```python
from build123d import *

# Parameters (mm, degrees)
EXTRUDE_1_DEPTH     = 4.8
SKETCH_2_R          = 2
CUT_EXTRUDE_1_DEPTH = 10
CHAMFER_1_SIZE      = 1
CHAMFER_2_SIZE      = 0.75
SKETCH_3_R          = 1.5
EXTRUDE_2_DEPTH     = 1.5
CHAMFER_3_SIZE      = 0.5
FILLET_2_R          = 0.2


with BuildPart() as part:
    # 스케치1 → 보스-돌출1 (new body)
    with BuildSketch(Plane.XY):
        Polygon((0, 0), (20.5, 0), (20.657326787, 1), (21.5, -1.146107212), (21.5, -2.146107212), (16, -2.146107212), (16, -6.5), (5, -6.5), (5, -2), (0, -2), align=None)
    extrude(amount=EXTRUDE_1_DEPTH)

    # 스케치2 → 컷-돌출1 (cut)
    with BuildSketch(Plane.XY.offset(4.8)):
        with Locations((10.5, -3.5)):
            Circle(SKETCH_2_R)
    extrude(amount=-CUT_EXTRUDE_1_DEPTH, mode=Mode.SUBTRACT)

    # 모따기1
    chamfer_1_edges = [part.edges().sort_by_distance(p)[0] for p in [
        (16, -6.5, 2.4),
        (5, -6.5, 2.4),
    ]]
    chamfer(chamfer_1_edges, length=CHAMFER_1_SIZE)

    # 모따기2
    chamfer_2_edges = [part.edges().sort_by_distance(p)[0] for p in [
        (21.5, -2.146107212, 2.4),
        (0, -2, 2.4),
    ]]
    chamfer(chamfer_2_edges, length=CHAMFER_2_SIZE)

    # 스케치3 → 보스-돌출2 (add)
    with BuildSketch(Plane(origin=(0, 0, 0), x_dir=(1, 0, 0), z_dir=(0, 1, 0))):
        with Locations(Location((2.5, -2.4, 0), (0, 0, 90))):
            Circle(SKETCH_3_R)
    extrude(amount=EXTRUDE_2_DEPTH)

    # 모따기3
    chamfer_3_edges = [part.edges().sort_by_distance(p)[0] for p in [
        (2.5, 1.5, 3.9),
    ]]
    chamfer(chamfer_3_edges, length=CHAMFER_3_SIZE)

    # 필렛2
    fillet_2_edges = [part.edges().sort_by_distance(p)[0] for p in [
        (8.5, -3.5, 0),
        (8.5, -3.5, 4.8),
    ]]
    fillet(fillet_2_edges, radius=FILLET_2_R)


solid = part.part
```
Verification items for the finished model (mm, model axes). A direction names the side the tool comes from. Coordinates: 2 decimals unless noted, no trailing zeros. Order: outer loops, then holes, each group sorted by start corner. A loop starts at its lowest first (then second) coordinate and runs counter-clockwise, first axis right, second up. Notation, with made-up numbers: (19.5, 74.25) -> (44.5, 74.25) arc R12 ccw to (44.5, 87.25) -> close; hole circle Ø5 at (-1, 38). An arc over 180 degrees is marked (long way). Put each result on its own line as item: value. Start each with the question number.
1) Cross-section at B-B (y = -3.5). Enter the section's corners in (x, z).
2) Release check for a two-part mould opening along X. For faces 1 (the cylindrical face through (8.9, -4.7, 2.4)), 2 (the flat face through (15.5, -6, 2.4)), 3 (the flat face through (18, -2.146, 2)) record: pulls with the +X half, pulls with the -X half, needs draft (parallel to the pull), parting line crosses it, or undercut.
3) Material ranges on L1, parallel to Y at x = 10.5, z = 2.95; L2, parallel to Y at x = 4.5, z = 4.4; L3, parallel to Y at x = 12.25, z = 1.7, recorded low to high.
4) Cross-section at C-C (z = 2.4). Enter the section's corners in (x, y), plus the area to 3 significant figures.
5) Cross-section at A-A (x = 10.5). Enter the section's corners in (y, z), plus the area to 3 significant figures.
6) Cross-section at D-D (x = 2.5). Enter the section's corners in (y, z).
7) Go/stop test with flat-tipped pins: pin 1 (1.5 mm diameter, centred on x = 14.5, z = 3, fed in from +Y); pin 2 (2.5 mm diameter, centred on y = -3, z = 2.5, fed in from +X); pin 3 (1.5 mm diameter, centred on x = 16, z = 3, fed in from -Y). Record where each tip stops, or that it passes through.
8) Tool access check on faces 4 (the flat face through (20.578, 0.493, 2.366)), 5 (the cylindrical face through (3.075, 0.493, 1.014)), 6 (the flat face through (3, -2, 2)). Record the directions out of +Z, -Z, +X, -X, +Y, -Y that give a thin tool (end or side, any length) a straight path to the whole face; none if there is none.
Geometry check:
1. outline: (5, 0) -> (8.3, 0) arc R0.2 ccw to (8.5, 0.2) -> (8.5, 4.6) arc R0.2 ccw to (8.3, 4.8) -> (5, 4.8) -> close; (12.5, 0.2) arc R0.2 ccw to (12.7, 0) -> (16, 0) -> (16, 4.8) -> (12.7, 4.8) arc R0.2 ccw to (12.5, 4.6) -> close
2. face 1: undercut
2. face 2: pulls with the +X half
2. face 3: needs draft
3. L1: y = -6.5 to -5.5, -1.5 to 0
3. L2: y = -2 to 0
3. L3: y = -6.5 to -4.47, -2.53 to 0
4. outline: (0, -1.25) -> (0.75, -2) -> (5, -2) -> (5, -5.5) -> (6, -6.5) -> (15, -6.5) -> (16, -5.5) -> (16, -2.15) -> (20.75, -2.15) -> (21.5, -1.4) -> (21.5, -1.15) -> (20.66, 1) -> (20.5, 0) -> (4, 0) -> (4, 1) -> (3.5, 1.5) -> (1.5, 1.5) -> (1, 1) -> (1, 0) -> (0, 0) -> close; hole circle Ø4 at (10.5, -3.5)
4. area: 83.4 mm^2
5. outline: (-6.5, 0) -> (-5.7, 0) arc R0.2 ccw to (-5.5, 0.2) -> (-5.5, 4.6) arc R0.2 ccw to (-5.7, 4.8) -> (-6.5, 4.8) -> close; (-1.5, 0.2) arc R0.2 ccw to (-1.3, 0) -> (0, 0) -> (0, 4.8) -> (-1.3, 4.8) arc R0.2 ccw to (-1.5, 4.6) -> close
5. area: 12.0 mm^2
6. outline: (-2, 0) -> (0, 0) -> (0, 0.9) -> (1, 0.9) -> (1.5, 1.4) -> (1.5, 3.4) -> (1, 3.9) -> (0, 3.9) -> (0, 4.8) -> (-2, 4.8) -> close
7. pin 1: stops at y = 0
7. pin 2: stops at x = 21.15
7. pin 3: stops at y = -6.25
8. face 4: +Z, -Z, +Y
8. face 5: +Y
8. face 6: +Z, -Z, -X, -Y
